from build123d import *

# Parameters (mm, degrees)
F0_R     = 17.0561
F1_DEPTH = 5.08
F2_R     = 16.129
F3_DEPTH = 1.27
F4_R     = 5.07999
F5_R     = 14.605
F6_DEPTH = 3.4642005339


# Not quite as in the source:
# - a fillet or chamfer is up to 0.001 mm smaller than in the source, because OpenCascade refuses the exact size


with BuildPart() as f1:
    # F0 (on Front) → F1 (new body)
    with BuildSketch(Plane.XZ):
        Circle(F0_R)
    extrude(amount=-F1_DEPTH)

    # F2 (on face) → F3 (join)
    with BuildSketch(Plane(origin=(0, 5.08, 0), x_dir=(-1, 0, 0), z_dir=(0, 1, 0))):
        Circle(F2_R)
    extrude(amount=F3_DEPTH)

    # F4 (radius 5.08 in the source; OpenCascade refuses exactly that, so slightly less here)
    f4_edges = [f1.edges().sort_by_distance(p)[0] for p in [
        (-17.0561, 0, 0),
    ]]
    fillet(f4_edges, radius=F4_R)

    # F5 (on face) → F6 (join)
    with BuildSketch(Plane(origin=(0, 6.35, 0), x_dir=(-1, 0, 0), z_dir=(0, 1, 0))):
        Circle(F5_R)
    extrude(amount=F6_DEPTH)


solid = f1.part
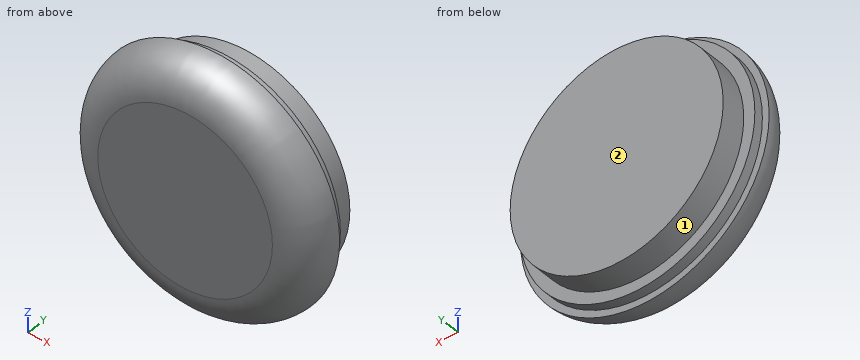
Verification items for the finished model (mm, model axes). Face numbers are marked on the shaded views. A direction names the side the tool comes from. Coordinates: 2 decimals unless noted, no trailing zeros. Loops run counter-clockwise (first coordinate to the right, second up) from the corner with the lowest first, then second, coordinate; pieces in that order, holes last. Notation, with made-up numbers: M 46,85.25 L 58,85.25 A26 ccw 58,115.25 Z; hole C 36,7.5 d7. An arc over 180 degrees is marked long. One line per item, written item: value.
1. Gauge pin test, flat ends, axial feed: P1, Ø3, axis at x = 9, y = 7.5, coming from the -Z side; P2, Ø1, axis at y = 7, z = 7, coming from the -X side; P3, Ø1, axis at x = 6.5, y = 8.5, coming from the -Z side. Record the tip position at first contact, or that the pin passes through.
Answers follow:
P1: z = -13.98
P2: x = -13.08
P3: z = -13.32
2. Section check D-D on y = 4.5. Record the cut outline in (x, z).
Answers follow:
outline: C 0,0 d34.05
3. Section check C-C on y = 8.75. Record the cut outline in (x, z) (3 decimals).
Answers follow:
outline: C 0,0 d29.21
4. Set-up check for the marked faces 1 and 2: record each of +Z, -Z, +X, -X, +Y, -Y from which the full face is reachable in a straight line by a thin tool's end or side.
Answers follow:
face 1: +Y
face 2: +Z, -Z, +X, -X, +Y
5. Material ranges on line 1 along Y through (x, z) = (7.5, 9.5); line 2 along Z through (x, y) = (-13, 4.75); line 3 along Z through (x, y) = (-10, 2.25), recorded low to high. Write a range as from..to.
Answers follow:
line 1: 0..9.81
line 2: -11.02..11.02
line 3: -12.74..12.74
